Could you check a few things on this model? Use its own coordinates, in mm. Face numbers are marked on the shaded views. Give positions to 0.01 mm unless a question says otherwise; leave off trailing zeros. Order: outer loops, then holes, each group sorted by start corner. A loop starts at its lowest first (then second) coordinate and runs counter-clockwise, first axis right, second up. Notation, with made-up numbers: (65.5, 25) - (75.5, 25) arc R22 cw to (75.5, 38) - close; hole circle Ø2 at (49.25, 36). An arc over 180 degrees is marked (long way). Put each result on its own line as item: value.
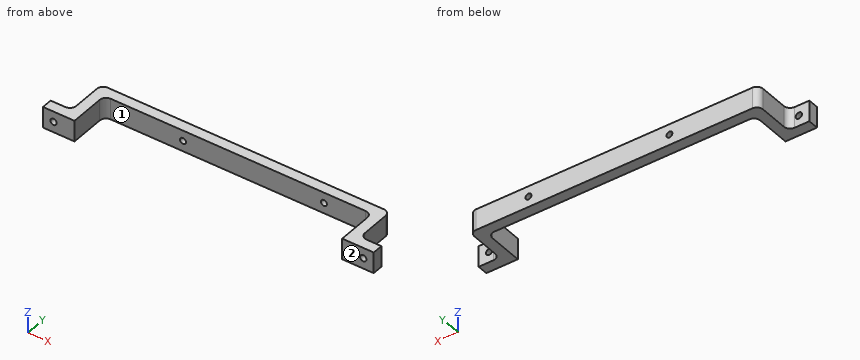
from build123d import *

# Parameters (mm, degrees)
BOSS_EXTRUDE1_DEPTH  = 10
SKETCH2_R            = 1.5
CUT_EXTRUDE1_DEPTH   = 10
FILLET1_R            = 3
FILLET1_OF_MIRROR1_R = 3
SKETCH3_R            = 1.425
CUT_EXTRUDE2_DEPTH   = 10


with BuildPart() as part:
    # Sketch1 → Boss-Extrude1 (new body)
    with BuildSketch(Plane.XY):
        Polygon((0, 0), (-68.64, 0), (-68.64, -19.5), (-78.64, -19.5), (-78.64, -24.5), (-63.64, -24.5), (-63.64, -5), (0, -5), align=None)
    boss_extrude1 = extrude(amount=BOSS_EXTRUDE1_DEPTH)

    # Sketch2 → Cut-Extrude1 (cut)
    with BuildSketch(Plane(origin=(0, -19.5, 0), x_dir=(1, 0, 0), z_dir=(0, 1, 0))):
        with Locations(Location((-73.64, -5, 0), (0, 0, 180))):
            Circle(SKETCH2_R)
    cut_extrude1 = extrude(amount=-CUT_EXTRUDE1_DEPTH, mode=Mode.SUBTRACT)

    # Fillet1
    fillet1_edges = [part.edges().sort_by_distance(p)[0] for p in [
        (-63.64, -5, 5),
        (-68.64, -19.5, 5),
        (-68.64, 0, 5),
    ]]
    fillet(fillet1_edges, radius=FILLET1_R)

    # Mirror1: Boss-Extrude1, Cut-Extrude1 across plane
    add(boss_extrude1.mirror(Plane(origin=(0, -5, 10), x_dir=(0, 0, 1), z_dir=(-1, 0, 0))))
    add(cut_extrude1.mirror(Plane(origin=(0, -5, 10), x_dir=(0, 0, 1), z_dir=(-1, 0, 0))), mode=Mode.SUBTRACT)

    # Fillet1 of Mirror1
    fillet1_of_mirror1_edges = [part.edges().sort_by_distance(p)[0] for p in [
        (63.64, -5, 5),
        (68.64, -19.5, 5),
        (68.64, 0, 5),
    ]]
    fillet(fillet1_of_mirror1_edges, radius=FILLET1_OF_MIRROR1_R)

    # Sketch3 → Cut-Extrude2 (cut)
    with BuildSketch(Plane(origin=(0, 0, 0), x_dir=(1, 0, 0), z_dir=(0, 1, 0))):
        with Locations(Location((40.788603054, -5, 0), (0, 0, 180))):
            Circle(SKETCH3_R)
        with Locations(Location((-26.211396946, -5, 0), (0, 0, 180))):
            Circle(SKETCH3_R)
    extrude(amount=-CUT_EXTRUDE2_DEPTH, mode=Mode.SUBTRACT)


solid = part.part
1) Suppose I cut it at D-D, the plane y = -14.75. List the corners of the cut face in (x, z) for me, and give its area (3 significant figures).
Filled in:
outline: (-68.64, 0) - (-63.64, 0) - (-63.64, 10) - (-68.64, 10) - close; (63.64, 0) - (68.64, 0) - (68.64, 10) - (63.64, 10) - close
area: 100 mm^2
2) Suppose I cut it at C-C, the plane x = -73.64. List the corners of the cut face in (y, z) for me, and give its area (3 significant figures).
Filled in:
outline: (-24.5, 0) - (-19.5, 0) - (-19.5, 3.5) - (-24.5, 3.5) - close; (-24.5, 6.5) - (-19.5, 6.5) - (-19.5, 10) - (-24.5, 10) - close
area: 35.0 mm^2
3) I'm going to push flat-ended pins straight in: pin 1 (2.5 mm diameter, centred on x = -73.64, z = 5, fed in from +Y); pin 2 (4 mm diameter, centred on x = 17.5, z = 4.5, fed in from +Y); pin 3 (3 mm diameter, centred on y = -6.5, z = 6.5, fed in from -X); pin 4 (1 mm diameter, centred on x = 4.5, z = 2.5, fed in from -Y). Where does each tip first touch, or does it pass through?
Filled in:
pin 1: passes through
pin 2: stops at y = 0
pin 3: stops at x = -68.64
pin 4: stops at y = -5
4) Suppose I cut it at B-B, the plane z = 5. State how many separate pieces and enclosed holes the cut face has, and give its area (3 significant figures).
Filled in:
separate pieces: 5
enclosed holes: 0
area: 927 mm^2
5) We'd pull the mould along X, two halves only. Please class the marked faces 1 and 2: pulls with the +X half, pulls with the -X half, needs draft (parallel to the pull), parting line crosses it, or undercut.
Filled in:
face 1: undercut
face 2: needs draft
6) If I drill on line 1 (X direction, y = -19.75, z = 4.75); line 2 (Z direction, x = -73.64, y = -21.75); line 3 (X direction, y = -8, z = 7.5), over which ranges is the centre line in solid material (lowest first)? Write a range as [from, to].
Filled in:
line 1: x = [-78.64, -75.12], [-72.16, -63.64], [63.64, 72.16], [75.12, 78.64]
line 2: z = [0, 3.5], [6.5, 10]
line 3: x = [-68.64, -63.64], [63.64, 68.64]
7) Suppose I cut it at A-A, the plane y = -21.5. List the corners of the cut face in (x, z) for me, and give its area (3 significant figures).
Filled in:
outline: (-78.64, 0) - (-63.64, 0) - (-63.64, 10) - (-78.64, 10) - close; (63.64, 0) - (78.64, 0) - (78.64, 10) - (63.64, 10) - close; hole circle Ø3 at (-73.64, 5); hole circle Ø3 at (73.64, 5)
area: 286 mm^2
